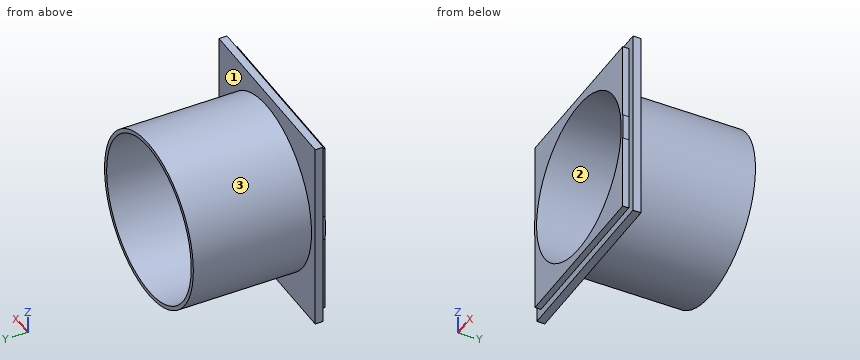
from build123d import *

# Parameters (mm, degrees)
CROQUIS1_W              = 41.5
CROQUIS1_H              = 44.4
SALIENTE_EXTRUIR1_DEPTH = 1.5
CROQUIS2_W              = 45.5
CROQUIS2_H              = 48.539759036
SALIENTE_EXTRUIR2_DEPTH = 2
CROQUIS3_R              = 21
SALIENTE_EXTRUIR3_DEPTH = 33
CROQUIS4_R              = 20
CORTAR_EXTRUIR1_DEPTH   = 72.653401873


with BuildPart() as part:
    # Croquis1 → Saliente-Extruir1 (new body)
    with BuildSketch(Plane(origin=(0, 0, 0), x_dir=(1, 0, 0), z_dir=(0, 1, 0))):
        with Locations((20.75, 22.2)):
            Rectangle(CROQUIS1_W, CROQUIS1_H)
    extrude(amount=SALIENTE_EXTRUIR1_DEPTH)

    # Croquis2 → Saliente-Extruir2 (add)
    with BuildSketch(Plane(origin=(0, 1.5, 0), x_dir=(1, 0, 0), z_dir=(0, 1, 0))):
        with Locations((20.75, 22.130120482)):
            Rectangle(CROQUIS2_W, CROQUIS2_H)
    extrude(amount=SALIENTE_EXTRUIR2_DEPTH)

    # Croquis3 → Saliente-Extruir3 (add)
    with BuildSketch(Plane.XZ):
        with Locations(Location((20.75, -22.2, 0), (0, 0, 270))):
            Circle(CROQUIS3_R)
    extrude(amount=-SALIENTE_EXTRUIR3_DEPTH)

    # Croquis4 → Cortar-Extruir1 (cut, through all)
    with BuildSketch(Plane(origin=(0, 33, 0), x_dir=(1, 0, 0), z_dir=(0, 1, 0))):
        with Locations(Location((20.75, 22.2, 0), (0, 0, 270))):
            Circle(CROQUIS4_R)
    extrude(amount=-CORTAR_EXTRUIR1_DEPTH, mode=Mode.SUBTRACT)


solid = part.part
The listing builds one solid part. Answer for the finished solid, in the listing's coordinates (mm). Face numbers are marked on the shaded views. Round coordinates to 2 decimals unless told otherwise and drop trailing zeros. Write each loop counter-clockwise with the first axis right and the second up, starting at its lowest first coordinate (ties: lowest second). Pieces come first, ordered by that corner, then holes. Notation, with made-up numbers: (-26.75, 81.5) - (-20.75, 81.5) arc R28 ccw to (-20.75, 108.5) - close; hole circle Ø11 at (1, -8.75). An arc over 180 degrees is marked (long way). Use one line per item in the form item = value. Start each with the question number.
Item 1: Determine the mould class of the marked faces 1, 2 and 3 for opening direction Z: +Z half, -Z half, draft (parallel to the pull), parting line (faces both ways), or undercut.
Item 2: Find the intervals of material crossed by line 1 (Z direction, x = 20, y = 15); line 2 (X direction, y = 21, z = -22.2); line 3 (Z direction, x = 13.5, y = 15), in increasing order. Write a range as [from, to].
Item 3: Flat-ended cylindrical pins translate along their axes: pin 1 Ø5 at (x, z) = (25.5, -37) entering from +Y (3 decimals); pin 2 Ø0.8 at (x, y) = (23.5, 0.5) entering from -Z; pin 3 Ø8 at (y, z) = (18, -3) entering from -X; pin 4 Ø10 at (x, y) = (19, 23) entering from +Z. Find the tip coordinate at first contact, or state that the pin passes through.
Item 4: A cutting plane is placed at A-A (x = 20.75). Write down the section's boundary in (y, z).
Item 5: A cutting plane is placed at C-C (y = 20). Write down the section's boundary in (x, z), plus the area to 3 significant figures.
Item 6: A cutting plane is placed at B-B (z = -22.2). Write down the section's boundary in (x, y).
The answers:
q1.face_1 = draft
q1.face_2 = undercut
q1.face_3 = parting line
q2.line_1 = [-43.19, -42.19], [-2.21, -1.21]
q2.line_2 = [-0.25, 0.75], [40.75, 41.75]
q2.line_3 = [-41.91, -40.84], [-3.56, -2.49]
q3.pin_1 = through
q3.pin_2 = -44.4
q3.pin_3 = 6.26
q3.pin_4 = -1.2
q4.outline = (0, -44.4) - (1.5, -44.4) - (1.5, -46.4) - (3.5, -46.4) - (3.5, -43.2) - (33, -43.2) - (33, -42.2) - (0, -42.2) - close; (0, -2.2) - (33, -2.2) - (33, -1.2) - (3.5, -1.2) - (3.5, 2.14) - (1.5, 2.14) - (1.5, 0) - (0, 0) - close
q5.outline = circle Ø42 at (20.75, -22.2); hole circle Ø40 at (20.75, -22.2)
q5.area = 129 mm^2
q6.outline = (-2, 1.5) - (-0.25, 1.5) - (-0.25, 0) - (0.75, 0) - (0.75, 33) - (-0.25, 33) - (-0.25, 3.5) - (-2, 3.5) - close; (40.75, 0) - (41.75, 0) - (41.75, 1.5) - (43.5, 1.5) - (43.5, 3.5) - (41.75, 3.5) - (41.75, 33) - (40.75, 33) - close
